Source: CAD feature listing. Evaluate the final solid. Frame: model axes, mm. A direction names the side the tool comes from. Give positions to 0.01 mm unless a question says otherwise; leave off trailing zeros. Write each loop counter-clockwise with the first axis right and the second up, starting at its lowest first coordinate (ties: lowest second). Pieces come first, ordered by that corner, then holes. Notation, with made-up numbers: (-24, 49.5) -> (31, 49.5) arc R14 cw to (31, 57.5) -> close; hole circle Ø10 at (20, 82.5). An arc over 180 degrees is marked (long way). Use a Markdown table: item, result. Add a question column.
```python
from build123d import *

# Parameters (mm, degrees)
SKETCH2_W           = 100
SKETCH2_H           = 4
BOSS_EXTRUDE1_DEPTH = 5
BOSS_EXTRUDE2_DEPTH = 4


with BuildPart() as part:
    # Sketch2 → Boss-Extrude1 (new body)
    with BuildSketch(Plane(origin=(0, 0, 0), x_dir=(1, 0, 0), z_dir=(0, 1, 0))):
        Rectangle(SKETCH2_W, SKETCH2_H)
    extrude(amount=BOSS_EXTRUDE1_DEPTH)

    # Sketch3 → Boss-Extrude2 (add)
    with BuildSketch(Plane.XY.offset(2)):
        Polygon((-50, 5), (-46, 5), (-47.4, 7), (-48.6, 7), align=None)
        Polygon((-42.6, 7), (-44, 5), (-40, 5), (-41.4, 7), align=None)
        Polygon((-36.6, 7), (-38, 5), (-34, 5), (-35.4, 7), align=None)
        Polygon((-30.6, 7), (-32, 5), (-28, 5), (-29.4, 7), align=None)
        Polygon((-24.6, 7), (-26, 5), (-22, 5), (-23.4, 7), align=None)
        Polygon((-18.6, 7), (-20, 5), (-16, 5), (-17.4, 7), align=None)
        Polygon((-12.6, 7), (-14, 5), (-10, 5), (-11.4, 7), align=None)
        Polygon((-6.6, 7), (-8, 5), (-4, 5), (-5.4, 7), align=None)
        Polygon((-0.6, 7), (-2, 5), (2, 5), (0.6, 7), align=None)
        Polygon((5.4, 7), (4, 5), (8, 5), (6.6, 7), align=None)
        Polygon((11.4, 7), (10, 5), (14, 5), (12.6, 7), align=None)
        Polygon((17.4, 7), (16, 5), (20, 5), (18.6, 7), align=None)
        Polygon((23.4, 7), (22, 5), (26, 5), (24.6, 7), align=None)
        Polygon((29.4, 7), (28, 5), (32, 5), (30.6, 7), align=None)
        Polygon((35.4, 7), (34, 5), (38, 5), (36.6, 7), align=None)
        Polygon((41.4, 7), (40, 5), (44, 5), (42.6, 7), align=None)
        Polygon((47.4, 7), (46, 5), (50, 5), (48.6, 7), align=None)
    extrude(amount=-BOSS_EXTRUDE2_DEPTH)


solid = part.part
```
(1) First-contact query: pin 1 Ø1.6 at (x, z) = (-15.5, 0) entering from +Y; pin 2 Ø0.6 at (x, z) = (-39, -1) entering from +Y; pin 3 Ø2 at (x, z) = (45.5, 0) entering from +Y. Flat tips, straight axial feed; report the tip coordinate or a pass-through.
(2) Material intervals for L1, parallel to Y at x = -45, z = 1.3; L2, parallel to Y at x = -37, z = -0.25, sorted ascending.
(3) Access query for faces 1 (the flat face through (-1, 3, 2)), 2 (the flat face through (-40.7, 6, 0)). Directions: +Z, -Z, +X, -X, +Y, -Y. A direction counts if a zero-diameter tool reaches every point of the face in a straight line with its end or side. Return the directions, or none.
(4) Cut plane A-A on y = 6. Count the separate pieces of the cut face and the enclosed holes in it, then the cut area to 3 significant figures.
(5) Cut plane B-B on x = 15. Return the cut outline in (y, z), then the cut area to 3 significant figures.
Output:
| question | item | result |
|---|---|---|
| 1 | pin 1 | y = 5.43 |
| 1 | pin 2 | y = 5 |
| 1 | pin 3 | y = 5.71 |
| 2 | L1 | 0 to 5 |
| 2 | L2 | 0 to 6.43 |
| 3 | face 1 | +Z, +X, -X, +Y, -Y |
| 3 | face 2 | +Z, -Z, +Y |
| 4 | separate pieces | 17 |
| 4 | enclosed holes | 0 |
| 4 | area | 177 mm^2 |
| 5 | outline | (0, -2) -> (5, -2) -> (5, 2) -> (0, 2) -> close |
| 5 | area | 20.0 mm^2 |
